The drawing under review shows one solid part. Ordinate dimensions are in mm from its lowest x, y, z. A direction names the side the tool comes from. Round coordinates to 2 decimals unless told otherwise and drop trailing zeros. Order: outer loops, then holes, each group sorted by start corner. A loop starts at its lowest first (then second) coordinate and runs counter-clockwise, first axis right, second up. Notation, with made-up numbers: M -5.75,36 L 16.25,36 A18 ccw 16.25,41 Z; hole C -20,85.25 d6. An arc over 180 degrees is marked long. Answer as a JSON object with one key per item and string values. Group by question number.
1) Consider section D-D, the plane z = 15. Write out the cut boundary in (x, y).
2) Consider section B-B, the plane x = 42. Write out the cut boundary in (y, z).
3) Insertion check: pin 1 Ø6 at (x, y) = (60, 54.5) entering from +Z. The pin has a flat end and moves straight along its axis. Give the tip position at first contact, or say it passes through.
4) For the marked faces 1 and 2, list the 3-axis set-ups (+Z, -Z, +X, -X, +Y, -Y) from which the entire face can be reached by the end or side of a thin tool; tool diameter is ignored.
5) The part is to be moulded in two halves that separate along X. For the marked faces 3, 4 and 5, say which applies: +X half, -X half, draft (parallel to the pull), parting line (faces both ways), or undercut.
6) Consider section A-A, the plane z = 6. Write out the cut boundary in (x, y), then the cut area to 3 significant figures.
7) To check wall thickness, follow line 1 (X direction, y = 67, z = 2.75); line 2 (Y direction, x = 53.5, z = 6.5); line 3 (X direction, y = 1.4, z = 15). State the ranges of each line that lie inside material, in increasing order.
8) Consider section C-C, the plane y = 26. Write out the cut boundary in (x, z).
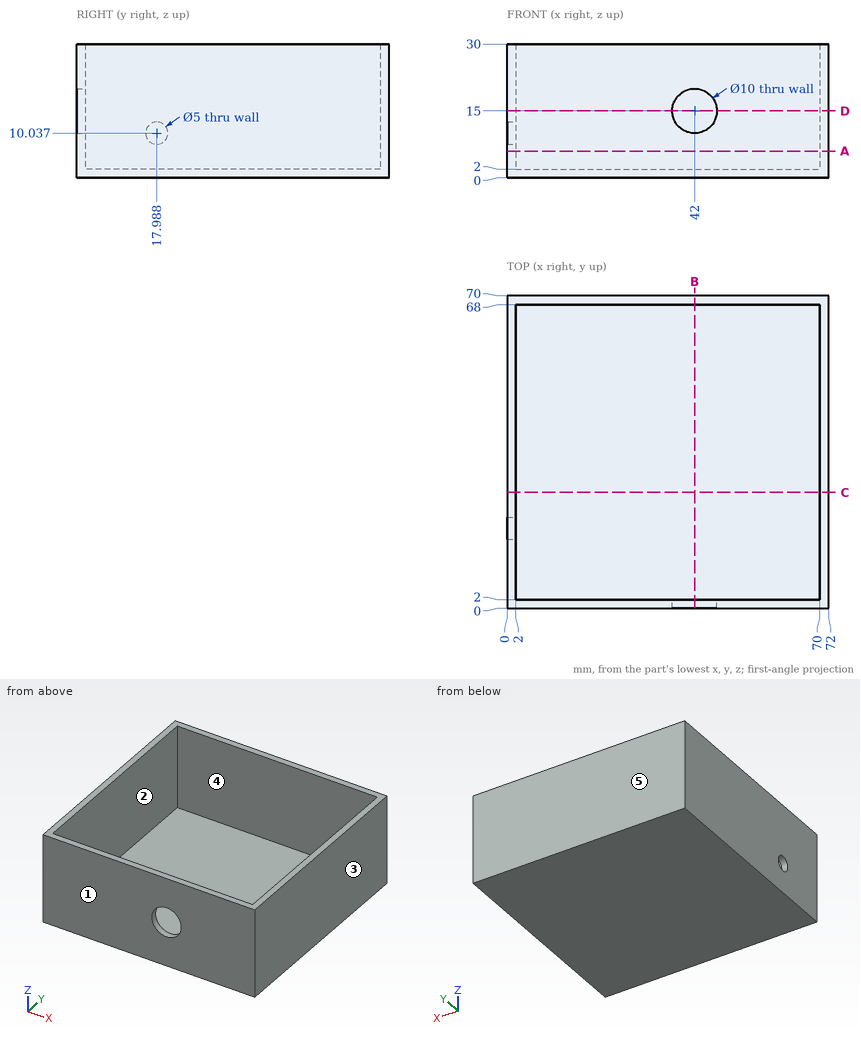
Results list:
{
 "1": {"outline": "M 0,0 L 37,0 L 37,2 L 2,2 L 2,68 L 70,68 L 70,2 L 47,2 L 47,0 L 72,0 L 72,70 L 0,70 Z"},
 "2": {"outline": "M 0,0 L 70,0 L 70,30 L 68,30 L 68,2 L 2,2 L 2,10 L 0,10 Z; M 0,20 L 2,20 L 2,30 L 0,30 Z"},
 "3": {"pin 1": "z = 2"},
 "4": {"face 1": "+Z, -Z, +X, -X, -Y", "face 2": "+Z"},
 "5": {"face 3": "+X half", "face 4": "undercut", "face 5": "draft"},
 "6": {"outline": "M 0,0 L 72,0 L 72,70 L 0,70 Z; hole M 2,2 L 70,2 L 70,68 L 2,68 Z", "area": "552 mm^2"},
 "7": {"line 1": "0 to 2, 70 to 72", "line 2": "0 to 2, 68 to 70", "line 3": "0 to 37, 47 to 72"},
 "8": {"outline": "M 0,0 L 72,0 L 72,30 L 70,30 L 70,2 L 2,2 L 2,30 L 0,30 Z"}
}
